Read the model definition and answer for the solid it produces. Units are mm, in the model's axes. Round coordinates to 2 decimals unless told otherwise and drop trailing zeros. Write each loop counter-clockwise with the first axis right and the second up, starting at its lowest first coordinate (ties: lowest second). Pieces come first, ordered by that corner, then holes. Notation, with made-up numbers: (31.25, 49.25) - (80.25, 49.25) arc R27 cw to (80.25, 72.25) - close; hole circle Ø4 at (18, 35.25). An arc over 180 degrees is marked (long way). One line per item, written item: value. Start each with the question number.
(1) A cutting plane is placed at A-A, the plane x = 235. Determine the outline of the cut face in (y, z).
(2) A cutting plane is placed at B-B, the plane y = -1. State how many separate pieces and enclosed holes the cut face has, plus the area to 3 significant figures.
(3) Find the intervals of material crossed by L1, parallel to Z at x = 239.5, y = -2.5; L2, parallel to Z at x = 230, y = -3.25; L3, parallel to Z at x = 255, y = -2, in increasing order.
(4) Flat-ended cylindrical pins translate along their axes: pin 1 Ø3 at (x, y) = (214.5, -2) entering from -Z; pin 2 Ø1.8 at (y, z) = (-2.5, -375.5) entering from -X; pin 3 Ø3 at (y, z) = (-2.5, -327.5) entering from +X; pin 4 Ø20 at (x, z) = (240.19, -32.55) entering from -Y. Find the tip coordinate at first contact, or state that the pin passes through.
from build123d import *

# Parameters (mm, degrees)
F0_R     = 16.5575031532
F0_W     = 25.0224173069
F0_H     = 73.3505785465
F1_DEPTH = 6


# Not quite as in the source:
# - a feature names something its author has since deleted; it is built from what else it names


with BuildPart() as f1:
    # F0 (on Front) → F1 (new body)
    with BuildSketch(Plane.XZ):
        with BuildLine():
            add(Edge.make_bspline(
                [(248.9335625079, 167.3540463153), (272.5197521804, 160.3214966928), (276.1214780845, -32.6489303119), (276.7706038072, -92.8803390196)],
                knots=[0, 0, 0, 0, 236.7397799676, 236.7397799676, 236.7397799676, 236.7397799676], degree=3))
            Line((248.9335625079, 167.3540463153), (221.9335625079, 167.3540463153))
            Line((221.9335625079, 167.3540463153), (221.9335625079, 147.3540463153))
            Line((221.9335625079, 147.3540463153), (211.9335625079, 147.3540463153))
            Line((211.9335625079, 147.3540463153), (211.9335625079, -105.6459536847))
            Line((211.9335625079, -105.6459536847), (244.4335625079, -105.6459536847))
            Line((244.4335625079, -105.6459536847), (244.4335625079, -110.6459536847))
            Line((244.4335625079, -110.6459536847), (276.9335625079, -110.6459536847))
            add(Edge.make_bspline(
                [(276.7706038072, -92.8803390196), (276.8875933326, -103.7356227789), (276.9086779216, -110.279341705), (276.9335625079, -110.6459536847)],
                knots=[236.7397799676, 236.7397799676, 236.7397799676, 236.7397799676, 279.4065138826, 279.4065138826, 279.4065138826, 279.4065138826], degree=3))
        make_face()
        with Locations((240.1929050684, -32.5540304184)):
            Circle(F0_R, mode=Mode.SUBTRACT)
        with Locations((234.4716570738, 97.3541972034)):
            Rectangle(F0_W, F0_H, mode=Mode.SUBTRACT)
        with BuildLine():
            add(Edge.make_bspline(
                [(276.7706038072, -128.4115683497), (276.8875933326, -117.5562845905), (276.9086779216, -111.0125656644), (276.9335625079, -110.6459536847)],
                knots=[236.7397799677, 236.7397799677, 236.7397799677, 236.7397799677, 279.4065138826, 279.4065138826, 279.4065138826, 279.4065138826], degree=3))
            Line((276.9335625079, -110.6459536847), (244.4335625079, -110.6459536847))
            Line((244.4335625079, -110.6459536847), (244.4335625079, -115.6459536847))
            Line((244.4335625079, -115.6459536847), (211.9335625079, -115.6459536847))
            Line((211.9335625079, -115.6459536847), (211.9335625079, -368.6459536847))
            Line((211.9335625079, -368.6459536847), (221.9335625079, -368.6459536847))
            Line((221.9335625079, -368.6459536847), (221.9335625079, -388.6459536847))
            Line((221.9335625079, -388.6459536847), (248.9335625079, -388.6459536847))
            add(Edge.make_bspline(
                [(248.9335625079, -388.6459536847), (272.5197521804, -381.6134040622), (276.1214780845, -188.6429770574), (276.7706038072, -128.4115683497)],
                knots=[0, 0, 0, 0, 236.7397799677, 236.7397799677, 236.7397799677, 236.7397799677], degree=3))
        make_face()
        with Locations((234.4716570738, -318.6461045727)):
            Rectangle(F0_W, F0_H, mode=Mode.SUBTRACT)
        with Locations((240.1929050684, -188.737876951)):
            Circle(F0_R, mode=Mode.SUBTRACT)
    extrude(amount=F1_DEPTH)


solid = f1.part
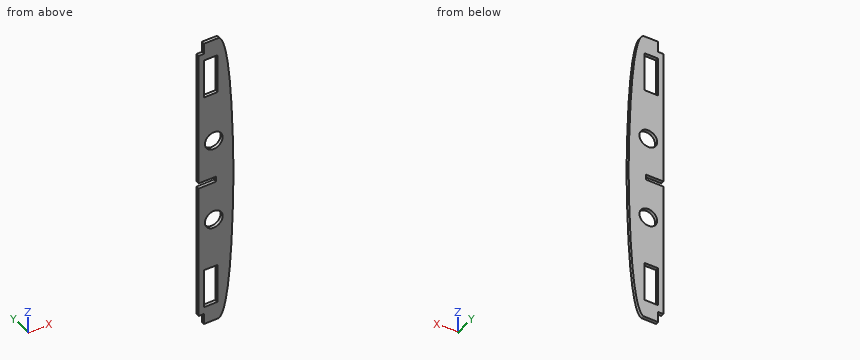
Here are the results:
1. outline: (-6, -388.65) - (0, -388.65) - (0, -355.32) - (-6, -355.32) - close; (-6, -281.97) - (0, -281.97) - (0, -204.46) - (-6, -204.46) - close; (-6, -173.02) - (0, -173.02) - (0, -115.65) - (-6, -115.65) - close; (-6, -105.65) - (0, -105.65) - (0, -48.28) - (-6, -48.28) - close; (-6, -16.83) - (0, -16.83) - (0, 60.68) - (-6, 60.68) - close; (-6, 134.03) - (0, 134.03) - (0, 167.35) - (-6, 167.35) - close
2. separate pieces: 1
2. enclosed holes: 4
2. area: 26,700 mm²
3. L1: -388.65 to -355.32, -281.97 to -205.28, -172.19 to -115.65, -105.65 to -49.1, -16.01 to 60.68, 134.03 to 167.35
3. L2: -388.65 to -355.32, -281.97 to -201.79, -175.69 to -115.65, -105.65 to -45.6, -19.51 to 60.68, 134.03 to 167.35
3. L3: -382.13 to -196.15, -181.33 to -39.96, -25.14 to 160.84
4. pin 1: z = -368.65
4. pin 2: x = 221.93
4. pin 3: x = 267.16
4. pin 4: through
